Solid Edge part; units mm, degrees
sketch "Sketch1" plane through (0, 0, 0) normal (0, 0, -1) x (-1, 0, 0)
  line L0 (1, -10.5) -> (1, 10.5)
  line L1 (1, 10.5) -> (-1, 10.5)
  line L2 (-1, 10.5) -> (-1, -10.5)
  line L3 (-1, -10.5) -> (1, -10.5)
revolve "RevolvedProtrusion1" add sketch "Sketch1" angle 360 about axis through (-1, -10.5, 0) along (0, 1, 0)
sketch "Sketch2" plane through (-1, 10.5, 0) normal (0, 1, 0) x (0, 0, 1)
  circle A0 centre (0, 0) radius 3.175
extrude "Protrusion1" add sketch "Sketch2" along normal blind 1
sketch "Sketch3" plane through (-1, -10.5, 0) normal (0, -1, 0) x (0, 0, 1)
  circle A0 centre (0, 0) radius 3.175
extrude "Protrusão_Extrudada_12" add sketch "Sketch3" along normal blind 1
For this review, take the finished solid that the model builds, in its own axes (mm). A direction names the side the tool comes from. Give positions to 0.01 mm unless a question says otherwise; leave off trailing zeros. Loops run counter-clockwise (first coordinate to the right, second up) from the corner with the lowest first, then second, coordinate; pieces in that order, holes last. Notation, with made-up numbers: M -14,-37.5 L 18,-37.5 A17 ccw 18,-30.5 Z; hole C -5.75,-30.75 d6. An arc over 180 degrees is marked long. One line per item, written item: value. Start each with the question number.
Q1. Draft analysis for pull direction Y (two halves, no side actions). For faces 1 (the face through (-3, -10.5, -1)), 2 (the face through (-1, 11.5, 0)), 3 (the face through (2.15, -10.99, -0.41)), state which applies: released by +Y, released by -Y, zero draft, split by the parting line, or undercut.
Q2. Add section D-D (y = 8.5). Give the boundary of the cut face in (x, z).
Q3. Clearance check with flat-ended pins moving along their axes: pin 1 Ø1.5 at (x, y) = (-0.5, 4) entering from +Z; pin 2 Ø3 at (y, z) = (3, -0.5) entering from -X; pin 3 Ø1 at (y, z) = (9, 2) entering from +X. State where each tip first meets the part, or that it passes through.
Q4. Add section A-A (z = 2.5). Give the boundary of the cut face in (x, y).
Q5. Machinability: for faces 4 (the face through (0.93, 10.99, -2.52)), 5 (the face through (-1, 0, -2)), which of the approach directions +Z, -Z, +X, -X, +Y, -Y give a long, thin tool a straight path to every point of the face, cutting with its end or side? Answer none if there is none.
Q6. Add section C-C (z = 0). Give the boundary of the cut face in (x, y) (3 decimals).
Q7. Add section B-B (x = -1). Give the boundary of the cut face in (y, z) (3 decimals).
Q8. For L1, parallel to Y at x = 1.25, z = -1.75; L2, parallel to Z at x = -1, y = -0.75; L3, parallel to X at y = -8.25, z = 0, list the stretches that pass through material, from the lowest coordinate up.
Reply:
1. face 1: undercut
1. face 2: released by +Y
1. face 3: zero draft
2. outline: C -1,0 d4
3. pin 1: z = 2
3. pin 2: x = -3
3. pin 3: x = 0.32
4. outline: M -2.96,-11.5 L 0.96,-11.5 L 0.96,-10.5 L -2.96,-10.5 Z; M -2.96,10.5 L 0.96,10.5 L 0.96,11.5 L -2.96,11.5 Z
5. face 4: +Y, -Y
5. face 5: none
6. outline: M -4.175,-11.5 L 2.175,-11.5 L 2.175,-10.5 L 1,-10.5 L 1,10.5 L 2.175,10.5 L 2.175,11.5 L -4.175,11.5 L -4.175,10.5 L -3,10.5 L -3,-10.5 L -4.175,-10.5 Z
7. outline: M -11.5,-3.175 L -10.5,-3.175 L -10.5,-2 L 10.5,-2 L 10.5,-3.175 L 11.5,-3.175 L 11.5,3.175 L 10.5,3.175 L 10.5,2 L -10.5,2 L -10.5,3.175 L -11.5,3.175 Z
8. L1: -11.5 to -10.5, 10.5 to 11.5
8. L2: -2 to 2
8. L3: -3 to 1
